The listing builds one solid part. Answer for the finished solid, in the listing's coordinates (mm). A direction names the side the tool comes from. Round coordinates to 2 decimals unless told otherwise and drop trailing zeros. Write each loop counter-clockwise with the first axis right and the second up, starting at its lowest first coordinate (ties: lowest second). Pieces come first, ordered by that corner, then holes. Notation, with made-up numbers: M 65,-5 L 72,-5 A17 ccw 72,22 Z; hole C 17,14 d10. An arc over 180 degrees is marked long. Put each result on its own line as item: value. Start each with the question number.
```python
from build123d import *

# Parameters (mm, degrees)
F1_DEPTH = 5


with BuildPart() as f1:
    # F0 (on Top) → F1 (new body)
    with BuildSketch(Plane.XY):
        Polygon((-357.880314, 85.929643), (-447.880314, 40.181844), (-447.880314, -138.234643), (-267.880314, -138.234643), (-267.880314, 40.181844), align=None)
        Polygon((-434.953884, -91.706066), (-357.880314, -54.201352), (-280.806743, -91.706066), (-280.806743, -113.134637), (-357.880314, -75.629924), (-434.953884, -113.134637), align=None, mode=Mode.SUBTRACT)
        Polygon((-434.953884, -35.636677), (-357.880314, 1.868036), (-280.806743, -35.636677), (-280.806743, -57.065249), (-357.880314, -19.560536), (-434.953884, -57.065249), align=None, mode=Mode.SUBTRACT)
        Polygon((-434.953884, 17.266547), (-357.880314, 54.77126), (-280.806743, 17.266547), (-280.806743, -4.162025), (-357.880314, 33.342688), (-434.953884, -4.162025), align=None, mode=Mode.SUBTRACT)
    extrude(amount=F1_DEPTH)


solid = f1.part
```
Item 1: Section C-C (z = 0.95) is taken. Give the vertices of the cut face in (x, y).
Item 2: Section D-D (y = -87) is taken. Give the vertices of the cut face in (x, z).
Item 3: A flat-ended cylindrical pin translates along its axis: pin 1 (3 mm diameter, centred on x = -371, z = 0.5, fed in from +Y). Find the tip coordinate at first contact, or state that the pin passes through.
Item 4: Section B-B (y = 50) is taken. Give the vertices of the cut face in (x, z), and give its area (3 significant figures).
Item 5: Determine the mould class of faces 3 (the flat face through (-359, -138.235, 2)), 4 (the flat face through (-434.954, -47, 2)), 5 (the flat face through (-447.88, -48, 2)), 6 (the flat face through (-312.25, 62.736, 2.465)) for opening direction Y: released by +Y, released by -Y, zero draft, split by the parting line, or undercut.
Item 6: Consider line 1 along Y through (x, z) = (-416.5, 3); line 2 along Y through (x, z) = (-378.5, 1.5); line 3 along X through (y, z) = (-39.5, 0.7). Determine where each line is inside the solid, lowest interval first. Write a range as [from, to].
Item 7: Which of the six approach directions +Z, -Z, +X, -X, +Y, -Y give full straight-line access (tool end or side, diameter ignored) to faces 1 (the flat face through (-280.807, -46, 2)), 2 (the flat face through (-267.88, -50, 2))?
Item 8: Section A-A (x = -370) is taken. Give the vertices of the cut face in (y, z), and give its area (3 significant figures).
Output values:
1. outline: M -447.88,-138.23 L -267.88,-138.23 L -267.88,40.18 L -357.88,85.93 L -447.88,40.18 Z; hole M -434.95,-113.13 L -357.88,-75.63 L -280.81,-113.13 L -280.81,-91.71 L -357.88,-54.2 L -434.95,-91.71 Z; hole M -434.95,-57.07 L -357.88,-19.56 L -280.81,-57.07 L -280.81,-35.64 L -357.88,1.87 L -434.95,-35.64 Z; hole M -434.95,-4.16 L -357.88,33.34 L -280.81,-4.16 L -280.81,17.27 L -357.88,54.77 L -434.95,17.27 Z
2. outline: M -447.88,0 L -425.28,0 L -425.28,5 L -447.88,5 Z; M -381.25,0 L -334.51,0 L -334.51,5 L -381.25,5 Z; M -290.48,0 L -267.88,0 L -267.88,5 L -290.48,5 Z
3. pin 1: stops at y = 80.02
4. outline: M -428.56,0 L -367.69,0 L -367.69,5 L -428.56,5 Z; M -348.08,0 L -287.2,0 L -287.2,5 L -348.08,5 Z
4. area: 609 mm^2
5. face 3: released by -Y
5. face 4: undercut
5. face 5: zero draft
5. face 6: released by +Y
6. line 1: y = [-138.23, -104.15], [-82.73, -48.09], [-26.66, 4.82], [26.25, 56.13]
6. line 2: y = [-138.23, -85.66], [-64.24, -29.59], [-8.17, 23.31], [44.74, 75.45]
6. line 3: x = [-447.88, -434.95], [-398.86, -316.9], [-280.81, -267.88]
7. face 1: +Z, -Z
7. face 2: +Z, -Z, +X, +Y, -Y
8. outline: M -138.23,0 L -81.53,0 L -81.53,5 L -138.23,5 Z; M -60.1,0 L -25.46,0 L -25.46,5 L -60.1,5 Z; M -4.03,0 L 27.45,0 L 27.45,5 L -4.03,5 Z; M 48.87,0 L 79.77,0 L 79.77,5 L 48.87,5 Z
8. area: 769 mm^2
